```python
from build123d import *

# Parameters (mm, degrees)
SKETCH1_W           = 140
SKETCH1_H           = 60
SKETCH1_W_2         = 132
SKETCH1_H_2         = 52
BOSS_EXTRUDE1_DEPTH = 150
BOSS_EXTRUDE3_DEPTH = 60
CUT_EXTRUDE1_DEPTH  = 4
SKETCH5_W           = 2.5
SKETCH5_H           = 4.1
CUT_EXTRUDE2_DEPTH  = 4


with BuildPart() as part:
    # Sketch1 → Boss-Extrude1 (new body)
    with BuildSketch(Plane(origin=(0, 0, 0), x_dir=(1, 0, 0), z_dir=(0, 1, 0))):
        with Locations((70, -30)):
            Rectangle(SKETCH1_W, SKETCH1_H)
        with Locations((70, -30)):
            Rectangle(SKETCH1_W_2, SKETCH1_H_2, mode=Mode.SUBTRACT)
    extrude(amount=BOSS_EXTRUDE1_DEPTH)

    # Sketch3 → Boss-Extrude3 (add)
    with BuildSketch(Plane.XY):
        Polygon((0, 0), (140, 6), (140, -4), (0, -4), align=None)
    extrude(amount=BOSS_EXTRUDE3_DEPTH)

    # Sketch4 → Cut-Extrude1 (cut)
    with BuildSketch(Plane.ZY):
        with BuildLine():
            Line((27, 0), (33, 0))
            Line((33, 0), (33, 2))
            add(Edge.make_bspline(
                [(33, 2), (33, 4.5), (30, 4.5), (27, 4.5), (27, 2)],
                knots=[3.141592654, 3.141592654, 3.141592654, 4.71238898, 4.71238898, 6.283185307, 6.283185307, 6.283185307], degree=2, weights=[1, 0.707106781, 1, 0.707106781, 1]))
            Line((27, 2), (27, 0))
        make_face()
    extrude(amount=-CUT_EXTRUDE1_DEPTH, mode=Mode.SUBTRACT)

    # Sketch5 → Cut-Extrude2 (cut)
    with BuildSketch(Plane.ZY):
        with Locations((39.75, 7)):
            Rectangle(SKETCH5_W, SKETCH5_H)
        with Locations((20.25, 7)):
            Rectangle(SKETCH5_W, SKETCH5_H)
    extrude(amount=-CUT_EXTRUDE2_DEPTH, mode=Mode.SUBTRACT)


solid = part.part
```
Check sheet for the modelled part. Datum: model origin and axes. Units: mm. A direction names the side the tool comes from. Round coordinates to 2 decimals unless told otherwise and drop trailing zeros. Order: outer loops, then holes, each group sorted by start corner. A loop starts at its lowest first (then second) coordinate and runs counter-clockwise, first axis right, second up. Notation, with made-up numbers: (78, 13.25) - (87, 13.25) arc R30 ccw to (87, 41.25) - close; hole circle Ø6 at (73.25, -36). An arc over 180 degrees is marked (long way). Answer as CSV lines item,"result". Start each with the question number.
1) Section check C-C (x = 85.5). Record the cut outline in (y, z).
2) Tool access check on faces 1 (the face through (140, 72, 30)), 2 (the face through (69.08, 2.96, 29.64)), 3 (the face through (2, 7, 41)). Record the directions out of +Z, -Z, +X, -X, +Y, -Y that give a thin tool (end or side, any length) a straight path to the whole face; none if there is none.
3) Scan lines: probe 1 along X at (y, z) = (27.5, 29.5); probe 2 along Z at (x, y) = (128, 91.5); probe 3 along Y at (x, z) = (77, 25.5). Record each from-to range of solid material in increasing order.
4) Section check B-B (z = 46.5). Record the cut outline in (x, y).
5) Draft check along Z on faces 4 (the face through (71, -4, 30)), 5 (the face through (4, 74, 30)), 6 (the face through (69, 72, 0)), 7 (the face through (69, 72, 60)). Enter one of: +Z half, -Z half, draft (parallel to the pull), parting line (faces both ways), or undercut.
6) Section check A-A (y = 129). Record the cut outline in (x, z).
7) Depth check by flat-ended pin: pin 1 (3 mm diameter, centred on x = 75.5, z = 39, fed in from +Y); pin 2 (2 mm diameter, centred on x = 91.5, z = 33.5, fed in from +Y). Enter the tip coordinate at first touch or a pass-through.
Determined:
1,outline,"(-4, 0) - (150, 0) - (150, 4) - (3.66, 4) - (3.66, 56) - (150, 56) - (150, 60) - (-4, 60) - close"
2,face 1,"+Z, -Z, +X, +Y, -Y"
2,face 2,"+Y"
2,face 3,"-X"
3,probe 1,"0 to 4, 136 to 140"
3,probe 2,"0 to 4, 56 to 60"
3,probe 3,"-4 to 3.3"
4,outline,"(0, -4) - (140, -4) - (140, 150) - (136, 150) - (136, 5.83) - (4, 0.17) - (4, 150) - (0, 150) - close"
5,face 4,"draft"
5,face 5,"undercut"
5,face 6,"-Z half"
5,face 7,"+Z half"
6,outline,"(0, 0) - (140, 0) - (140, 60) - (0, 60) - close; hole (4, 4) - (136, 4) - (136, 56) - (4, 56) - close"
7,pin 1,"y = 3.3"
7,pin 2,"y = 3.96"
